Geometry check sheet. Reference: the model listing, model coordinates, mm. Give positions to 0.01 mm unless a question says otherwise; leave off trailing zeros. Order: outer loops, then holes, each group sorted by start corner. A loop starts at its lowest first (then second) coordinate and runs counter-clockwise, first axis right, second up. Notation, with made-up numbers: M -28.5,53.25 L 26.5,53.25 A14 cw 26.5,69.25 Z; hole C -35.5,31 d4. An arc over 180 degrees is marked long. Use CSV: the item, a comma, the result in double quotes. Start each with the question number.
from build123d import *

# Parameters (mm, degrees)
SKETCH_1_W          = 37.5
SKETCH_1_H          = 36.5
EXTRUDE_1_DEPTH     = 1
CUT_EXTRUDE_1_DEPTH = 1
CUT_EXTRUDE_2_DEPTH = 1
FILLET_1_R          = 2
SKETCH_4_W          = 13
SKETCH_4_H          = 6
CUT_EXTRUDE_3_DEPTH = 1


with BuildPart() as part:
    # 草图1 → 凸台-拉伸1 (new body)
    with BuildSketch(Plane(origin=(0, 0, 0), x_dir=(1, 0, 0), z_dir=(0, 1, 0))):
        Rectangle(SKETCH_1_W, SKETCH_1_H)
    extrude(amount=EXTRUDE_1_DEPTH)

    # 草图2 → 切除-拉伸1 (cut)
    with BuildSketch(Plane(origin=(0, 1, 0), x_dir=(1, 0, 0), z_dir=(0, 1, 0))):
        Polygon((-11.75, 18.25), (-18.75, 13.25), (-18.75, 18.25), align=None)
        Polygon((18.75, 18.25), (11.75, 18.25), (18.75, 13.25), align=None)
        Polygon((11.75, -18.25), (18.75, -13.25), (18.75, -18.25), align=None)
        Polygon((-18.75, -18.25), (-11.75, -18.25), (-18.75, -13.25), align=None)
    extrude(amount=-CUT_EXTRUDE_1_DEPTH, mode=Mode.SUBTRACT)

    # 草图3 → 切除-拉伸2 (cut)
    with BuildSketch(Plane(origin=(0, 1, 0), x_dir=(1, 0, 0), z_dir=(0, 1, 0))):
        with BuildLine():
            Line((-11.5, 16.25), (11.5, 16.25))
            ThreePointArc((11.5, 16.25), (12.5, 15.25), (11.5, 14.25))
            Line((11.5, 14.25), (-11.5, 14.25))
            ThreePointArc((-11.5, 14.25), (-12.5, 15.25), (-11.5, 16.25))
        make_face()
        with BuildLine():
            Line((-11.5, -16.25), (11.5, -16.25))
            ThreePointArc((11.5, -16.25), (12.5, -15.25), (11.5, -14.25))
            Line((11.5, -14.25), (-11.5, -14.25))
            ThreePointArc((-11.5, -14.25), (-12.5, -15.25), (-11.5, -16.25))
        make_face()
    extrude(amount=-CUT_EXTRUDE_2_DEPTH, mode=Mode.SUBTRACT)

    # 圆角1
    fillet_1_edges = [part.edges().sort_by_distance(p)[0] for p in [
        (-18.75, 0.5, 13.25),
        (-11.75, 0.5, 18.25),
        (11.75, 0.5, 18.25),
        (18.75, 0.5, 13.25),
        (18.75, 0.5, -13.25),
        (11.75, 0.5, -18.25),
        (-11.75, 0.5, -18.25),
        (-18.75, 0.5, -13.25),
    ]]
    fillet(fillet_1_edges, radius=FILLET_1_R)

    # 草图4 → 切除-拉伸3 (cut)
    with BuildSketch(Plane(origin=(0, 1, 0), x_dir=(1, 0, 0), z_dir=(0, 1, 0))):
        with Locations((12.25, 0)):
            Rectangle(SKETCH_4_W, SKETCH_4_H)
    extrude(amount=-CUT_EXTRUDE_3_DEPTH, mode=Mode.SUBTRACT)


solid = part.part
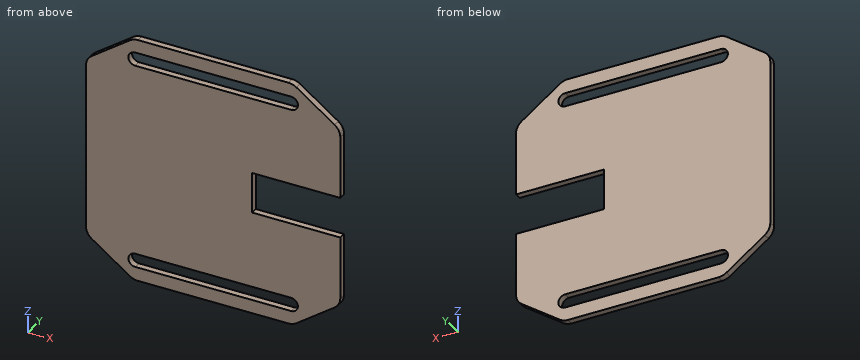
(1) Sectioned sample at B-B on z = -15.25. Record the cut outline in (x, y), then the cut area to 3 significant figures.
(2) Go/stop test with flat-tipped pins: P1, Ø0.5, axis at x = 13, y = 0.5, coming from the +Z side; P2, Ø8, axis at x = 1.5, z = 10.5, coming from the -Y side. Record where each tip stops, or that it passes through.
(3) Thickness scan on line 1 (Z direction, x = -11, y = 0.1); line 2 (Z direction, x = 6, y = 0.9); line 3 (Z direction, x = 12, y = 0.5). Record the ranges inside material, lowest first.
(4) Sectioned sample at A-A on x = -8. Record the cut outline in (y, z), then the cut area to 3 significant figures.
(5) Sectioned sample at C-C on x = 8.5. Record the cut outline in (y, z), then the cut area to 3 significant figures.
(6) Sectioned sample at D-D on y = 0.6. Record the cut outline in (x, z), then the cut area to 3 significant figures.
Responses:
1,outline,"M -15.95,0 L -12.5,0 L -12.5,1 L -15.95,1 Z; M 12.5,0 L 15.95,0 L 15.95,1 L 12.5,1 Z"
1,area,"6.90 mm2"
2,P1,"z = 17.54"
2,P2,"y = 0"
3,line 1,"-18.25 to -16.25, -14.25 to 14.25, 16.25 to 18.25"
3,line 2,"-18.25 to -16.25, -14.25 to -3, 3 to 14.25, 16.25 to 18.25"
3,line 3,"-18.04 to -16.12, -14.38 to -3, 3 to 14.38, 16.12 to 18.04"
4,outline,"M 0,-18.25 L 1,-18.25 L 1,-16.25 L 0,-16.25 Z; M 0,-14.25 L 1,-14.25 L 1,14.25 L 0,14.25 Z; M 0,16.25 L 1,16.25 L 1,18.25 L 0,18.25 Z"
4,area,"32.5 mm2"
5,outline,"M 0,-18.25 L 1,-18.25 L 1,-16.25 L 0,-16.25 Z; M 0,-14.25 L 1,-14.25 L 1,-3 L 0,-3 Z; M 0,3 L 1,3 L 1,14.25 L 0,14.25 Z; M 0,16.25 L 1,16.25 L 1,18.25 L 0,18.25 Z"
5,area,"26.5 mm2"
6,outline,"M -18.75,-12.22 A2 ccw -17.91,-13.85 L -12.27,-17.88 A2 ccw -11.11,-18.25 L 11.11,-18.25 A2 ccw 12.27,-17.88 L 17.91,-13.85 A2 ccw 18.75,-12.22 L 18.75,-3 L 5.75,-3 L 5.75,3 L 18.75,3 L 18.75,12.22 A2 ccw 17.91,13.85 L 12.27,17.88 A2 ccw 11.11,18.25 L -11.11,18.25 A2 ccw -12.27,17.88 L -17.91,13.85 A2 ccw -18.75,12.22 Z; hole M -11.5,-16.25 L 11.5,-16.25 A1 ccw 11.5,-14.25 L -11.5,-14.25 A1 ccw Z; hole M -11.5,14.25 L 11.5,14.25 A1 ccw 11.5,16.25 L -11.5,16.25 A1 ccw Z"
6,area,"1,120 mm2"
